```python
from build123d import *

# Parameters (mm, degrees)
F1_DEPTH = 40
F3_DEPTH = 4


with BuildPart() as f1:
    # F0 (on Top) → F1 (new body)
    with BuildSketch(Plane.XY):
        Polygon((120, -20.038911), (120, -15), (0, 0), (0, -5.038911), align=None)
    extrude(amount=F1_DEPTH)

    # F2 (on face) → F3 (join)
    with BuildSketch(Plane(origin=(0, 0, 0), x_dir=(1, 0, 0), z_dir=(0, 0, -1))):
        Polygon((0, 10.077822), (0, 5.038911), (120, 20.038911), (120, 25.077822), align=None)
    extrude(amount=-F3_DEPTH)


solid = f1.part
```
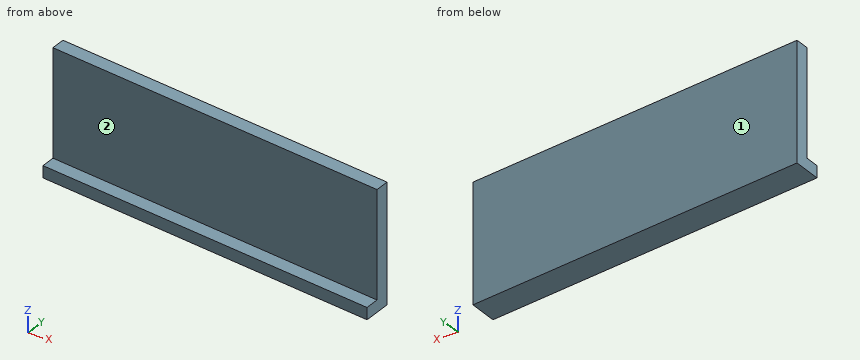
CAD build for the part. Positions are in the model's coordinates, mm. Face numbers are marked on the shaded views. A direction names the side the tool comes from. Round coordinates to 2 decimals unless told otherwise and drop trailing zeros. Order: outer loops, then holes, each group sorted by start corner. A loop starts at its lowest first (then second) coordinate and runs counter-clockwise, first axis right, second up. Notation, with made-up numbers: (31, 44.5) - (44, 44.5) arc R6 cw to (44, 53.5) - close; hole circle Ø5 at (68.5, 18.25). An arc over 180 degrees is marked (long way). Use CSV: the item, a comma, the result in double quotes. Start each with the question number.
1) Pin check, flat tips, straight feed: pin 1 Ø1 at (y, z) = (-5.5, 8) entering from -X; pin 2 Ø6 at (x, z) = (76, 24.5) entering from -Y; pin 3 Ø1 at (x, z) = (78, 32.5) entering from +Y; pin 4 Ø5 at (x, z) = (46, 9) entering from -Y. Stop position of each tip, or through.
2) Saw through at C-C (y = -21.75). List the corners of the cut face in (x, z), and give its area (3 significant figures).
3) Saw through at A-A (x = 100). List the corners of the cut face in (y, z), and give its area (3 significant figures).
4) Tool access for the marked faces 1 and 2: list every direction of +Z, -Z, +X, -X, +Y, -Y with a clear straight run to the whole face (end or side of a thin tool).
5) Saw through at B-B (z = 11). List the corners of the cut face in (x, y).
6) Wall check: L1, parallel to Z at x = 68.5, y = -14.25; L2, parallel to Y at x = 91, z = 5 (3 decimals); L3, parallel to Y at x = 50, z = 32.5. Give the ranges that are in metal, low to high. Write a range as [from, to].
Values follow:
1,pin 1,"stops at x = 0"
1,pin 2,"stops at y = -14.91"
1,pin 3,"stops at y = -9.69"
1,pin 4,"stops at y = -11.1"
2,outline,"(93.38, 0) - (120, 0) - (120, 4) - (93.38, 4) - close"
2,area,"106 mm2"
3,outline,"(-22.58, 0) - (-12.5, 0) - (-12.5, 40) - (-17.54, 40) - (-17.54, 4) - (-22.58, 4) - close"
3,area,"222 mm2"
4,face 1,"+Z, -Z, +X, +Y"
4,face 2,"+Z, -X, -Y"
5,outline,"(0, -5.04) - (120, -20.04) - (120, -15) - (0, 0) - close"
6,L1,"z = [0, 4]"
6,L2,"y = [-16.414, -11.375]"
6,L3,"y = [-11.29, -6.25]"
